Part model, mm, in its own coordinate system. A direction names the side the tool comes from. Give positions to 0.01 mm unless a question says otherwise; leave off trailing zeros. Order: outer loops, then holes, each group sorted by start corner. A loop starts at its lowest first (then second) coordinate and runs counter-clockwise, first axis right, second up. Notation, with made-up numbers: (7, -22.75) - (49, -22.75) arc R10 cw to (49, -13.75) - close; hole circle Ø10 at (42, 26). An arc over 180 degrees is marked (long way). One line per item, written item: value.
```python
from build123d import *

# Parameters (mm, degrees)
SKETCH1_R           = 4
BOSS_EXTRUDE1_DEPTH = 54.002621
SKETCH2_R           = 2.165
CUT_EXTRUDE1_DEPTH  = 9
SKETCH4_R           = 3.5
CUT_EXTRUDE2_DEPTH  = 55.298094693


with BuildPart() as part:
    # Sketch1 → Boss-Extrude1 (new body)
    with BuildSketch(Plane.XY):
        Circle(SKETCH1_R)
    extrude(amount=BOSS_EXTRUDE1_DEPTH)

    # Sketch2 → Cut-Extrude1 (cut, symmetric)
    with BuildSketch(Plane(origin=(0, 0, 0), x_dir=(0, 0, -1), z_dir=(1, 0, 0))):
        with Locations(Location((-46.502621, 0, 0), (0, 0, 180))):
            Circle(SKETCH2_R)
    extrude(amount=CUT_EXTRUDE1_DEPTH, both=True, mode=Mode.SUBTRACT)

    # Sketch4 → Cut-Extrude2 (cut, through all)
    with BuildSketch(Plane(origin=(0, 0, 0), x_dir=(0, 0, -1), z_dir=(1, 0, 0))):
        with Locations((-46.502621, 0)):
            Circle(SKETCH4_R)
    extrude(amount=-CUT_EXTRUDE2_DEPTH, mode=Mode.SUBTRACT)


solid = part.part
```
1) Slice it at C-C on x = 3.5. Write the cut outline in (y, z) (1 decimal), then the cut area to 3 significant figures.
Answer:
outline: (-1.9, 0) - (1.9, 0) - (1.9, 45.5) arc R2.2 cw to (-1.9, 45.5) - close; (-1.9, 47.5) arc R2.2 cw to (1.9, 47.5) - (1.9, 54) - (-1.9, 54) - close
area: 195 mm2
2) Slice it at B-B on x = -1.25. Write the cut outline in (y, z), then the cut area to 3 significant figures.
Answer:
outline: (-3.8, 0) - (3.8, 0) - (3.8, 54) - (-3.8, 54) - close; hole circle Ø7 at (0, 46.5)
area: 372 mm2
3) Two-plate mould, pull along Z, no slides. Class faces 3 (the face through (0, 0, 0)), 4 (the face through (0, 0, 54.003)), 5 (the face through (2.028, -0.65, 48.568)): pulls with the +Z half, pulls with the -Z half, needs draft (parallel to the pull), parting line crosses it, or undercut.
Answer:
face 3: pulls with the -Z half
face 4: pulls with the +Z half
face 5: undercut
4) Slice it at D-D on z = 37.5. Write the cut outline in (x, y), then the cut area to 3 significant figures.
Answer:
outline: circle Ø8 at (0, 0)
area: 50.3 mm2
5) Slice it at A-A on y = -1.25. Write the cut outline in (x, z), then the cut area to 3 significant figures.
Answer:
outline: (-3.8, 0) - (3.8, 0) - (3.8, 44.73) - (0, 44.73) - (0, 43.23) - (-3.8, 43.23) - close; (-3.8, 49.77) - (0, 49.77) - (0, 48.27) - (3.8, 48.27) - (3.8, 54) - (-3.8, 54) - close
area: 372 mm2
6) Wall check: line 1 along Z through (x, y) = (-1.85, 0); line 2 along Z through (x, y) = (-1, -0.75); line 3 along X through (y, z) = (-0.25, 39.5). Give the ranges that are in metal, low to high. Write a range as [from, to].
Answer:
line 1: z = [0, 43], [50, 54]
line 2: z = [0, 43.08], [49.92, 54]
line 3: x = [-3.99, 3.99]
7) Drop flat-ended pins along their axis: P1, Ø1.5, axis at x = 2.5, z = 37.5, coming from the -Y side; P2, Ø1, axis at x = 2, z = 11.5, coming from the -Y side; P3, Ø2, axis at y = 2.5, z = 16, coming from the -X side. Give the stop position or say it passes through.
Answer:
P1: stops at y = -3.6
P2: stops at y = -3.71
P3: stops at x = -3.71
8) Which spindle directions (+Z, -Z, +X, -X, +Y, -Y) get a long thin tool onto all of the face, cutting with end or side? Do faces 1 (the face through (-1.528, -3.105, 44.888)), 2 (the face through (3.695, -1.532, 26.623)). Say none if no direction does.
Answer:
face 1: -X
face 2: +Z, -Z
